Check sheet for the modelled part. Datum: model origin and axes. Units: mm. A direction names the side the tool comes from. Give positions to 0.01 mm unless a question says otherwise; leave off trailing zeros. Order: outer loops, then holes, each group sorted by start corner. A loop starts at its lowest first (then second) coordinate and runs counter-clockwise, first axis right, second up.
Item 1: Access from +Z, -Z, +X, -X, +Y, -Y to the whole of each face (thin tool, end or side, straight path). Record for faces 5 (the flat face through (35.5, 0, 19)), 6 (the flat face through (0, 14, 19)), 7 (the flat face through (28.1, -9.44, 19.37)), 8 (the flat face through (0, -14, 19)).
Item 2: Sectioned sample at D-D on z = 7.25. Record the boundary of the cut face in (x, y).
Item 3: Sectioned sample at A-A on y = 18. Record the boundary of the cut face in (x, z).
Item 4: Sectioned sample at B-B on x = -23. Record the boundary of the cut face in (y, z), and give its area (3 significant figures).
Item 5: Sectioned sample at C-C on z = 26.75. Record the boundary of the cut face in (x, y).
Item 6: Material ranges on line 1 along Y through (x, z) = (-35.5, 6); line 2 along X through (y, z) = (20.5, 5.5); line 3 along X through (y, z) = (-19, 5.25), recorded low to high.
Item 7: Release check for a two-part mould opening along Y. For faces 1 (the cylindrical face through (-38.5, 18.1, 5.1)), 2 (the flat face through (-41.5, 0, 5)), 3 (the cylindrical face through (-38.5, -17.9, 5.1)), 4 (the flat face through (-1, -24, 5)) record: released by +Y, released by -Y, zero draft, split by the parting line, or undercut.
Item 8: Gauge pin test, flat ends, axial feed: P1, Ø5.5, axis at x = -8, z = 17, coming from the +Y side; P2, Ø5, axis at x = 35.5, y = -18, coming from the -Z side; P3, Ø4, axis at x = 23.5, z = 23.5, coming from the +Y side; P4, Ø12, axis at y = 0, z = 18, coming from the -X side. Record the tip position at first contact, or that the pin passes through.
from build123d import *

# Parameters (mm, degrees)
SKETCH1_W           = 83
SKETCH1_H           = 48
BOSS_EXTRUDE1_DEPTH = 10
BOSS_EXTRUDE2_DEPTH = 19
SKETCH3_R           = 5
SKETCH3_R_2         = 6
SKETCH3_R_3         = 3
CUT_EXTRUDE1_DEPTH  = 30


with BuildPart() as part:
    # Sketch1 → Boss-Extrude1 (new body)
    with BuildSketch(Plane.XY):
        Rectangle(SKETCH1_W, SKETCH1_H)
    extrude(amount=BOSS_EXTRUDE1_DEPTH)

    # Sketch2 → Boss-Extrude2 (add)
    with BuildSketch(Plane.XY.offset(10)):
        Polygon((-35.5, 5), (-20.5, 14), (20.5, 14), (35.5, 5), (35.5, -5), (20.5, -14), (-20.5, -14), (-35.5, -5), align=None)
    extrude(amount=BOSS_EXTRUDE2_DEPTH)

    # Sketch3 → Cut-Extrude1 (cut, through all)
    with BuildSketch(Plane.XY.offset(29)):
        Circle(SKETCH3_R)
        with Locations((-23, 0)):
            Circle(SKETCH3_R_2)
        with Locations((23, 0)):
            Circle(SKETCH3_R_2)
        with Locations((-35.5, 18)):
            Circle(SKETCH3_R_3)
        with Locations((35.5, 18)):
            Circle(SKETCH3_R_3)
        with Locations((35.5, -18)):
            Circle(SKETCH3_R_3)
        with Locations((-35.5, -18)):
            Circle(SKETCH3_R_3)
    extrude(amount=-CUT_EXTRUDE1_DEPTH, mode=Mode.SUBTRACT)


solid = part.part
Report:
1. face 5: +Z, +X, +Y, -Y
1. face 6: +Z, +X, -X, +Y
1. face 7: +Z, +X, -Y
1. face 8: +Z, +X, -X, -Y
2. outline: (-41.5, -24) - (41.5, -24) - (41.5, 24) - (-41.5, 24) - close; hole circle Ø6 at (-35.5, -18); hole circle Ø6 at (-35.5, 18); hole circle Ø12 at (-23, 0); hole circle Ø10 at (0, 0); hole circle Ø12 at (23, 0); hole circle Ø6 at (35.5, -18); hole circle Ø6 at (35.5, 18)
3. outline: (-41.5, 0) - (-38.5, 0) - (-38.5, 10) - (-41.5, 10) - close; (-32.5, 0) - (32.5, 0) - (32.5, 10) - (-32.5, 10) - close; (38.5, 0) - (41.5, 0) - (41.5, 10) - (38.5, 10) - close
4. outline: (-24, 0) - (-6, 0) - (-6, 29) - (-12.5, 29) - (-12.5, 10) - (-24, 10) - close; (6, 0) - (24, 0) - (24, 10) - (12.5, 10) - (12.5, 29) - (6, 29) - close
4. area: 607 mm2
5. outline: (-35.5, -5) - (-20.5, -14) - (20.5, -14) - (35.5, -5) - (35.5, 5) - (20.5, 14) - (-20.5, 14) - (-35.5, 5) - close; hole circle Ø12 at (-23, 0); hole circle Ø10 at (0, 0); hole circle Ø12 at (23, 0)
6. line 1: y = -24 to -21, -15 to 15, 21 to 24
6. line 2: x = -41.5 to -37.16, -33.84 to 33.84, 37.16 to 41.5
6. line 3: x = -41.5 to -38.33, -32.67 to 32.67, 38.33 to 41.5
7. face 1: undercut
7. face 2: zero draft
7. face 3: undercut
7. face 4: released by -Y
8. P1: stops at y = 14
8. P2: passes through
8. P3: stops at y = 13.4
8. P4: stops at x = -35.5
